Autodesk Inventor part; units mm, degrees
ref_plane "YZ Plane" through (0, 0, 0) normal (1, 0, 0) x (0, 1, 0)
ref_plane "XZ Plane" through (0, 0, 0) normal (0, 1, 0) x (-1, 0, 0)
ref_plane "XY Plane" through (0, 0, 0) normal (0, 0, 1) x (1, 0, 0)
sketch "Sketch1" plane through (0, 0, 0) normal (0, 1, 0) x (-1, 0, 0)
  line L0 (49.1429, 49.1429) -> (-36.8571, 49.1429)
  line L1 (-36.8571, 49.1429) -> (-36.8571, -36.8571)
  line L2 (-36.8571, -36.8571) -> (49.1429, -36.8571)
  line L3 (49.1429, -36.8571) -> (49.1429, 49.1429)
  line L4 (52.1429, 52.1429) -> (-39.8571, 52.1429)
  line L5 (-39.8571, 52.1429) -> (-39.8571, -39.8571)
  line L6 (-39.8571, -39.8571) -> (52.1429, -39.8571)
  line L7 (52.1429, -39.8571) -> (52.1429, 52.1429)
  point P0 (0, 0)
  dimension "d0" = 86
  dimension "d1" = 86
  dimension "d2" = 92
extrude "Extrusion1" add sketch "Sketch1" along normal blind 45 contours L3 L2 L1 L0 | L7 L6 L5 L4
shell "Shell1" thickness 3 removed faces 1 at (9.1905, 45, -9.1905)
sketch "Sketch3" plane through (-49.1429, 3, -36.8571) normal (0, 1, 0) x (1, 0, 0)
  line L0 (86, -86) -> (0, -86)
  line L1 (86, 0) -> (0, 0)
  line L2 (13, -86) -> (73, -86)
  line L3 (73, -86) -> (73, 0)
  line L4 (73, 0) -> (13, 0)
  line L5 (13, 0) -> (13, -86)
  line L6 (86, 0) -> (86, -86)
  line L7 (86, -73) -> (0, -73)
  line L8 (0, -73) -> (0, -13)
  line L9 (0, -13) -> (86, -13)
  line L10 (86, -13) -> (86, -73)
  line L11 (0, -86) -> (0, 0)
  point P0 (49.1429, -36.8571)
  point P1 (73, -73)
  point P2 (73, -13)
  point P3 (13, 0)
  point P4 (13, -13)
  point P5 (13, -73)
  point P6 (73, -86)
  dimension "d6" = 13
  dimension "d7" = 13
  dimension "d8" = 13
  dimension "d9" = 13
extrude "Extrusion2" cut sketch "Sketch3" against normal blind 40 contours L0 L5 L7 L3 | L7 L3 L9 L6 | L7 L5 L9 L3 | L7 L8 L9 L5 | L9 L5 L1 L3
sketch "Sketch4" plane through (-49.1429, 3, 36.1429) normal (0, 1, 0) x (1, 0, 0)
  line L0 (86, -13) -> (0, -13)
  line L1 (0, -13) -> (0, 73)
  line L2 (0, 73) -> (86, 73)
  line L3 (86, 73) -> (86, -13)
  line L4 (89, -16) -> (89, 76)
  line L5 (89, 76) -> (-3, 76)
  line L6 (-3, 76) -> (-3, -16)
  line L7 (-3, -16) -> (89, -16)
  line L8 (8.2, 64.8) -> (8.2, -4.8)
  line L9 (8.2, -4.8) -> (77.8, -4.8)
  line L10 (77.8, -4.8) -> (77.8, 64.8)
  line L11 (77.8, 64.8) -> (8.2, 64.8)
  circle A0 centre (8.2, -4.8) radius 2.4
  circle A1 centre (8.2, 64.8) radius 2.4
  circle A2 centre (77.8, -4.8) radius 2.4
  circle A3 centre (77.8, 64.8) radius 2.4
  point P0 (49.1429, 36.1429)
  dimension "d12" = 69.6
  dimension "d13" = 4.8
  dimension "d14" = 4.8
  dimension "d15" = 4.8
  dimension "d16" = 4.8
extrude "Extrusion3" cut sketch "Sketch4" against normal blind 25 contours L11 A1 L8 | L8 A1 L11 | A0 L9 L8 | L8 L9 A0 | A3 L10 L11 | L11 L10 A3 | A2 L10 L9 | L9 L10 A2
fillet "Fillet1" radius 5 4 edges at (-36.1429, 1.5, 36.1429) (-36.1429, 1.5, -23.8571) (23.8571, 1.5, 36.1429) (23.8571, 1.5, -23.8571)
sketch "Sketch5" plane through (39.8571, 0, 52.1429) normal (1, 0, 0) x (0, 0, -1)
  line L0 (0, 0) -> (92, 0)
  line L1 (92, 0) -> (92, 45)
  line L2 (0, 45) -> (92, 45)
  line L3 (0, 0) -> (0, 45)
  point P0 (52.1429, 0)
extrude "Extrusion4" add sketch "Sketch5" along normal blind 4
sketch "Sketch6" plane through (0, 45, 0) normal (0, 1, 0) x (1, 0, 0)
  line L0 (-52.1429, 39.8571) -> (-52.1429, -52.1429)
  line L1 (-52.1429, -52.1429) -> (43.8571, -52.1429)
  line L2 (43.8571, -52.1429) -> (43.8571, -56.1429)
  line L3 (43.8571, -56.1429) -> (-52.1429, -56.1429)
  line L4 (-52.1429, -56.1429) -> (-52.1429, -52.1429)
  line L5 (-52.1429, 39.8571) -> (43.8571, 39.8571)
  line L6 (43.8571, 39.8571) -> (43.8571, 43.8571)
  line L7 (43.8571, 43.8571) -> (-52.1429, 43.8571)
  line L8 (-52.1429, 43.8571) -> (-52.1429, 39.8571)
  line L9 (43.8571, 39.8571) -> (43.8571, -52.1429)
  line L10 (-52.1429, -56.1429) -> (-56.1429, -56.1429)
  line L11 (-56.1429, -56.1429) -> (-56.1429, 43.8571)
  line L12 (-56.1429, 43.8571) -> (-52.1429, 43.8571)
  line L13 (-52.1429, 43.8571) -> (-52.1429, -56.1429)
  point P0 (0, 0)
  dimension "d22" = 4
  dimension "d23" = 4
  dimension "d26" = 4
extrude "Extrusion5" add sketch "Sketch6" against normal up to surface (45 mm away) contours L8 L7 L6 L5 | L0 L4 L10 L11 L12 L8 | L1 L2 L3 L4
sketch "Sketch7" plane through (-49.1429, 3, -36.8571) normal (0, 1, 0) x (1, 0, 0)
  arc A0 (8, -13) -> (13, -8) centre (8, -8) ccw
  line L0 (13, -8) -> (13, 0)
  line L1 (13, 0) -> (0, 0)
  line L2 (0, 0) -> (0, -13)
  line L3 (0, -13) -> (8, -13)
  circle A1 centre (8.2, -8.2) radius 2.4
  arc A2 (13, -78) -> (8, -73) centre (8, -78) ccw
  line L4 (8, -73) -> (0, -73)
  line L5 (0, -73) -> (0, -86)
  line L6 (0, -86) -> (13, -86)
  line L7 (13, -86) -> (13, -78)
  circle A3 centre (8.2, -77.8) radius 2.4
  arc A4 (78, -73) -> (73, -78) centre (78, -78) ccw
  line L8 (73, -78) -> (73, -86)
  line L9 (73, -86) -> (86, -86)
  line L10 (86, -86) -> (86, -73)
  line L11 (86, -73) -> (78, -73)
  circle A5 centre (77.8, -77.8) radius 2.4
  arc A6 (73, -8) -> (78, -13) centre (78, -8) ccw
  line L12 (78, -13) -> (86, -13)
  line L13 (86, -13) -> (86, 0)
  line L14 (86, 0) -> (73, 0)
  line L15 (73, 0) -> (73, -8)
  circle A7 centre (77.8, -8.2) radius 2.4
  point P0 (49.1429, -36.8571)
extrude "Extrusion6" add sketch "Sketch7" along normal blind 2
properties part number "BigMotorDerzavka"
Source: CAD feature listing. Evaluate the final solid. Frame: model axes, mm. A direction names the side the tool comes from. Give positions to 0.01 mm unless a question says otherwise; leave off trailing zeros. Loops run counter-clockwise (first coordinate to the right, second up) from the corner with the lowest first, then second, coordinate; pieces in that order, holes last. Notation, with made-up numbers: (59, 54) -> (75, 54) arc R20 ccw to (75, 85) -> close; hole circle Ø10 at (71.25, 76). An arc over 180 degrees is marked (long way). Put each result on its own line as item: value. Start each with the question number.
1) Contact query for flat-ended pins moving along their axis: P1, Ø4, axis at x = 31.5, z = -29.5, coming from the +Y side; P2, Ø4, axis at x = 28.66, z = -28.66, coming from the +Y side. Output: stop coordinate, or through.
2) Reachability of faces 5 (the face through (-49.143, 23, 7)), 6 (the face through (23.857, 3, -33)) from +Z, -Z, +X, -X, +Y, -Y: full face, straight path, thin tool, end or side. Return the list, or none.
3) Cut plane B-B (x = -15.5). Return loops of the section in (y, z).
4) Cut plane A-A (z = 23). Return loops of the section in (x, y), then the cut area to 3 significant figures.
5) Cut plane C-C (y = 11). Return loops of the section in (x, z).
6) Cut plane D-D (z = 45.5). Return loops of the section in (x, y), then the cut area to 3 significant figures.
7) Draft query along X for faces 1 (the face through (-7, 0, -38)), 2 (the face through (-56.143, 23, 7)), 3 (the face through (43.857, 23, 7)), 4 (the face through (-37.57, 2.46, -25.36)). Return one class per face: released by +X, released by -X, zero draft, split by the parting line, or undercut.
8) Material intervals for probe 1 along X at (y, z) = (24.5, 3); probe 2 along Z at (x, y) = (33, 13); probe 3 along X at (y, z) = (3, -30), sorted ascending.
Results are:
1. P1: stops at y = 5
1. P2: passes through
2. face 5: +Y
2. face 6: +Y, -Y
3. outline: (0, -43.86) -> (45, -43.86) -> (45, -36.86) -> (0, -36.86) -> close; (0, 49.14) -> (45, 49.14) -> (45, 56.14) -> (0, 56.14) -> close
4. outline: (-56.14, 0) -> (-49.14, 0) -> (-49.14, 45) -> (-56.14, 45) -> close; (36.86, 0) -> (43.86, 0) -> (43.86, 45) -> (36.86, 45) -> close
4. area: 630 mm2
5. outline: (-56.14, -43.86) -> (43.86, -43.86) -> (43.86, 56.14) -> (-56.14, 56.14) -> close; hole (-49.14, -36.86) -> (36.86, -36.86) -> (36.86, 49.14) -> (-49.14, 49.14) -> close
6. outline: (-56.14, 0) -> (-36.14, 0) -> (-36.14, 5) -> (-49.14, 5) -> (-49.14, 45) -> (-56.14, 45) -> close; (23.86, 0) -> (43.86, 0) -> (43.86, 45) -> (36.86, 45) -> (36.86, 5) -> (23.86, 5) -> close
6. area: 760 mm2
7. face 1: zero draft
7. face 2: released by -X
7. face 3: released by +X
7. face 4: undercut
8. probe 1: x = -56.14 to -49.14, 36.86 to 43.86
8. probe 2: z = -43.86 to -36.86, 49.14 to 56.14
8. probe 3: x = -56.14 to -42.93, -38.95 to -36.14, 23.86 to 26.67, 30.65 to 43.86
